For this review, take the finished solid that the model builds, in its own axes (mm). Round coordinates to 2 decimals unless told otherwise and drop trailing zeros. Write each loop counter-clockwise with the first axis right and the second up, starting at its lowest first coordinate (ties: lowest second). Pieces come first, ordered by that corner, then holes.
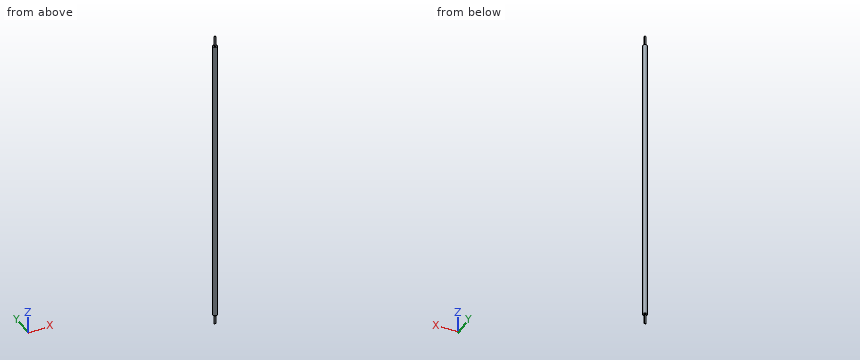
from build123d import *

# Parameters (mm, degrees)
ESQUISSE1_R             = 0.875
BOSS_EXTRU_1_DEPTH      = 122
ESQUISSE2_W             = 0.62970299
ESQUISSE2_H             = 8
BOSS_EXTRU_2_DEPTH      = 0.25
CONG_1_R                = 0.3
ENL_V_MAT_EXTRU_1_DEPTH = 0.06


with BuildPart() as part:
    # Esquisse1 → Boss.-Extru.1 (new body)
    with BuildSketch(Plane.XY):
        Circle(ESQUISSE1_R)
    extrude(amount=BOSS_EXTRU_1_DEPTH)

    # Esquisse2 → Boss.-Extru.2 (add)
    with BuildSketch(Plane(origin=(0, 0, 0), x_dir=(1, 0, 0), z_dir=(0, 1, 0))):
        Rectangle(ESQUISSE2_W, ESQUISSE2_H)
        with Locations((0, -122)):
            Rectangle(ESQUISSE2_W, ESQUISSE2_H)
    extrude(amount=BOSS_EXTRU_2_DEPTH)

    # Congé1
    cong_1_edges = [part.edges().sort_by_distance(p)[0] for p in [
        (-0.875, 0, 0),
        (-0.875, 0, 122),
    ]]
    fillet(cong_1_edges, radius=CONG_1_R)

    # Esquisse3 → Enlèv. mat.-Extru.1 (cut)
    with BuildSketch(Plane.XZ):
        Polygon((-0.023732379, -2.988428768), (-0.023732379, -2.840992871), (0.021139416, -2.840992871), (0.021139416, -2.988428768), (0.168575313, -2.988428768), (0.168575313, -3.033300563), (0.021139416, -3.033300563), (0.021139416, -3.18073646), (-0.023732379, -3.18073646), (-0.023732379, -3.033300563), (-0.171168277, -3.033300563), (-0.171168277, -2.988428768), align=None)
    extrude(amount=-ENL_V_MAT_EXTRU_1_DEPTH, mode=Mode.SUBTRACT)


solid = part.part
(1) For line 1 along Z through (x, y) = (0.1, 0.4); line 2 along X through (y, z) = (0.15, 61); line 3 along X through (y, z) = (0.65, 59), list the stretches that pass through material, from the lowest coordinate up.
Geometry check:
line 1: z = 0 to 122
line 2: x = -0.86 to 0.86
line 3: x = -0.59 to 0.59
(2) For pin 1 Ø0.7 at (x, z) = (0, -1) entering from +Y, flat-tipped, find the tip position at first contact; note if it passes through.
Geometry check:
pin 1: stops at y = 0.25
(3) We need section A-A, the plane z = 84.5. Give the boundary of the cut face in (x, y) (3 decimals), and give its area (3 significant figures).
Geometry check:
outline: circle Ø1.75 at (0, 0)
area: 2.41 mm2
